For this review, take the finished solid that the model builds, in its own axes (mm). A direction names the side the tool comes from. Give positions to 0.01 mm unless a question says otherwise; leave off trailing zeros. Write each loop counter-clockwise with the first axis right and the second up, starting at its lowest first coordinate (ties: lowest second). Pieces come first, ordered by that corner, then holes.
1) Draft analysis for pull direction X (two halves, no side actions). For faces 1 (the face through (-1, 1, 21.59)), 2 (the face through (-34.637, 1.524, 9.658)), 3 (the face through (-29.227, -22.41, 10.644)), state which applies: pulls with the +X half, pulls with the -X half, needs draft (parallel to the pull), parting line crosses it, or undercut.
2) Machinability: for faces 4 (the face through (0, 0, 19.05)), 5 (the face through (27, -22, 0)), which of the approach directions +Z, -Z, +X, -X, +Y, -Y give a long, thin tool a straight path to every point of the face, cutting with its end or side? Answer none if there is none.
3) For P1, Ø1.5, axis at y = -13, z = 3, coming from the +X side; P2, Ø12, axis at y = -20, z = 3, coming from the -X side; P3, Ø4, axis at y = 26.5, z = 17.5, coming from the +X side, all flat-tipped, find the tip position at first contact; note any pin that passes through.
4) We need section C-C on z = 4.25. Give the boundary of the cut face in (x, y), and give its area (3 significant figures).
5) Wall thickness on line 1 along Y through (x, z) = (0, 12.75); line 2 along Z through (x, y) = (2, -33.5): over which ranges is each line inside the solid? List them lowest first.
6) We need section A-A on x = 0. Give the boundary of the cut face in (y, z), and give its area (3 significant figures).
from build123d import *

# Parameters (mm, degrees)
F0_R     = 36.83
F1_DEPTH = 19.05
F2_R     = 34.671
F3_DEPTH = 97.79
F4_R     = 36.83
F5_DEPTH = 2.54


with BuildPart() as f1:
    # F0 (on Top) → F1 (new body)
    with BuildSketch(Plane.XY):
        Circle(F0_R)
    extrude(amount=F1_DEPTH)

    # F2 (on face) → F3 (cut)
    with BuildSketch(Plane.XY.offset(19.05)):
        Circle(F2_R)
    extrude(amount=-F3_DEPTH, mode=Mode.SUBTRACT)

    # F4 (on face) → F5 (join)
    with BuildSketch(Plane.XY.offset(19.05)):
        Circle(F4_R)
    extrude(amount=F5_DEPTH)


solid = f1.part
Results list:
1. face 1: needs draft
1. face 2: undercut
1. face 3: parting line crosses it
2. face 4: -Z
2. face 5: -Z, +X, -X, +Y, -Y
3. P1: stops at x = 34.73
3. P2: stops at x = -34.07
3. P3: stops at x = 27.5
4. outline: circle Ø73.66 at (0, 0); hole circle Ø69.34 at (0, 0)
4. area: 485 mm2
5. line 1: y = -36.83 to -34.67, 34.67 to 36.83
5. line 2: z = 19.05 to 21.59
6. outline: (-36.83, 0) - (-34.67, 0) - (-34.67, 19.05) - (34.67, 19.05) - (34.67, 0) - (36.83, 0) - (36.83, 21.59) - (-36.83, 21.59) - close
6. area: 269 mm2
